CAD build for the part. Positions are in the model's coordinates, mm. A direction names the side the tool comes from. Coordinates: 2 decimals unless noted, no trailing zeros. Order: outer loops, then holes, each group sorted by start corner. A loop starts at its lowest first (then second) coordinate and runs counter-clockwise, first axis right, second up. Notation, with made-up numbers: M 10,-14 L 50,-14 A8 cw 50,-5 Z; hole C -29.75,-24.5 d4. An arc over 180 degrees is marked long. One line per item, written item: value.
from build123d import *

# Parameters (mm, degrees)
L_ANGLE_L2X1_5X0_1875_1_DEPTH = 600
CUT_EXTRUDE1_REACH            = 308.647
M8_CLEARANCE_HOLE1_D          = 9


with BuildPart() as part:
    # Sketch14 → L angle L2X1.5X0.1875(1) (new body)
    with BuildSketch(Plane(origin=(0, 300, 0), x_dir=(0, 0, 1), z_dir=(0, -1, 0))):
        with BuildLine():
            Line((0, 0), (0, 50.8))
            Line((0, 50.8), (0.00508, 50.8))
            ThreePointArc((0.00508, 50.8), (3.369083943, 49.406583943), (4.7625, 46.04258))
            Line((4.7625, 46.04258), (4.7625, 9.525))
            ThreePointArc((4.7625, 9.525), (6.157403955, 6.157403955), (9.525, 4.7625))
            Line((9.525, 4.7625), (33.34258, 4.7625))
            ThreePointArc((33.34258, 4.7625), (36.706583943, 3.369083943), (38.1, 0.00508))
            Line((38.1, 0.00508), (38.1, 0))
            Line((38.1, 0), (0, 0))
        make_face()
    extrude(amount=L_ANGLE_L2X1_5X0_1875_1_DEPTH)

    # Sketch15 → Cut-Extrude1 (cut, up to next)
    with BuildSketch(Plane.XY, mode=Mode.PRIVATE) as cut_extrude1_sk1:
        Polygon((-50.8, -300), (0, -300), (0, -249.2), (-48.3, -297.5), (-50.8, -295), align=None)
    cut_extrude1_tool1 = extrude(cut_extrude1_sk1.sketch, amount=CUT_EXTRUDE1_REACH, mode=Mode.PRIVATE) & part.part
    # Sketch15 → Cut-Extrude1 (cut, up to next)
    with BuildSketch(Plane.XY, mode=Mode.PRIVATE) as cut_extrude1_sk2:
        Polygon((-50.8, 300), (0, 300), (0, 249.2), (-47.264466094, 296.464466094), (-50.8, 295), align=None)
    cut_extrude1_tool2 = extrude(cut_extrude1_sk2.sketch, amount=CUT_EXTRUDE1_REACH, mode=Mode.PRIVATE) & part.part
    add(cut_extrude1_tool1.solids().sort_by_distance((-17.092568, -283.136241, 0))[0], mode=Mode.SUBTRACT)
    add(cut_extrude1_tool2.solids().sort_by_distance((-17.155727, 283.162516, 0))[0], mode=Mode.SUBTRACT)

    # M8 Clearance Hole1 (through all)
    with Locations(Plane.XY.offset(4.7625)):
        with Locations((-40.8, 275.857864376), (-20.00508, 255.062944376), (-20.00508, -255.062944376), (-40.8, -275.857864376)):
            Hole(M8_CLEARANCE_HOLE1_D / 2)


solid = part.part
Q1. Slice it at C-C (z = 27.5). List the corners of the cut face in (x, y).
Recorded:
outline: M -4.76,-253.96 L 0,-249.2 L 0,249.2 L -4.76,253.96 Z
Q2. Drill centre lines: line 1 along Z through (x, y) = (-9, 195.5); line 2 along X through (y, z) = (188.5, 23); line 3 along Y through (x, z) = (-40, 2). Where is each one in solid material? Low to high.
Recorded:
line 1: z = 0 to 4.79
line 2: x = -4.76 to 0
line 3: y = -289.2 to -280.29, -271.43 to 271.43, 280.29 to 289.2
Q3. Pin check, flat tips, straight feed: pin 1 Ø1 at (x, y) = (-38, 72) entering from +Z; pin 2 Ø7 at (y, z) = (83, 24) entering from -X; pin 3 Ø10.5 at (x, y) = (-40.8, 275.86) entering from -Z; pin 4 Ø6 at (x, z) = (-42.5, 4.5) entering from -Y. Stop position of each tip, or through.
Recorded:
pin 1: stops at z = 4.76
pin 2: stops at x = -4.76
pin 3: stops at z = 0
pin 4: stops at y = -294.7
Q4. Which spindle directions (+Z, -Z, +X, -X, +Y, -Y) get a long thin tool onto all of the face, cutting with end or side? Do faces 5 (the face through (-4.762, 4, 21)), 6 (the face through (0, 3, 19)). Say none if no direction does.
Recorded:
face 5: +Z, -X, +Y, -Y
face 6: +Z, -Z, +X, +Y, -Y
Q5. Slice it at B-B (x = -30.5). List the corners of the cut face in (y, z).
Recorded:
outline: M -279.7,0 L 279.7,0 L 279.7,4.76 L -279.7,4.76 Z
Q6. Mould opens along Y. For faces 1 (the face through (-13, 262.2, 3.4)), 2 (the face through (-43.22, 279.65, 2.35)), 3 (the face through (-28, 4, 4.762)), 4 (the face through (-13.3, -262.5, 3.4)) say: released by +Y, released by -Y, zero draft, split by the parting line, or undercut.
Recorded:
face 1: released by +Y
face 2: undercut
face 3: zero draft
face 4: released by -Y
